from build123d import *

# Parameters (mm, degrees)
SKETCH1_R           = 1.5
BOSS_EXTRUDE1_DEPTH = 0.5
SKETCH2_R           = 1.5
BOSS_EXTRUDE2_DEPTH = 0.5
BOSS_EXTRUDE6_DEPTH = 10.25


with BuildPart() as part:
    # Sketch1 → Boss-Extrude1 (new, symmetric)
    with BuildSketch(Plane(origin=(0, 0, 0), x_dir=(0, 0, -1), z_dir=(1, 0, 0))):
        Polygon((0, 0), (0, 6), (14, 6), (14, -0.7), (9.85, -1), (9.7, 0), align=None)
        with Locations((10.4, 4)):
            Circle(SKETCH1_R, mode=Mode.SUBTRACT)
    extrude(amount=BOSS_EXTRUDE1_DEPTH, both=True)



with BuildPart() as body_2:
    # Sketch2 → Boss-Extrude2 (new, symmetric)
    with BuildSketch(Plane.ZY.offset(11.5)):
        Polygon((-9.7, 0), (-9.85, -1), (-14, -0.7), (-14, 6), (0, 6), (0, 0), align=None)
        with Locations(Location((-10.4, 4, 0), (0, 0, 180))):
            Circle(SKETCH2_R, mode=Mode.SUBTRACT)
    extrude(amount=BOSS_EXTRUDE2_DEPTH, both=True)


with BuildPart() as part_1:
    add(part.part)

    add(body_2.part)  # Boss-Extrude6 merges body 2
    # Sketch9 → Boss-Extrude6 (add)
    with BuildSketch(Plane.XY):
        with BuildLine():
            Line((-11, 6), (-12, 6))
            ThreePointArc((-12, 6), (-11.414213562, 7.414213562), (-10, 8))
            Line((-10, 8), (-1.5, 8))
            ThreePointArc((-1.5, 8), (-0.085786438, 7.414213562), (0.5, 6))
            Line((0.5, 6), (-0.5, 6))
            ThreePointArc((-0.5, 6), (-0.792893219, 6.707106781), (-1.5, 7))
            Line((-1.5, 7), (-10, 7))
            ThreePointArc((-10, 7), (-10.707106781, 6.707106781), (-11, 6))
        make_face()
    extrude(amount=-BOSS_EXTRUDE6_DEPTH)


solid = part_1.part
Input: part model. Units: mm. Frame: model coordinates. A direction names the side the tool comes from. Round coordinates to 2 decimals unless told otherwise and drop trailing zeros. Loops run counter-clockwise (first coordinate to the right, second up) from the corner with the lowest first, then second, coordinate; pieces in that order, holes last. Notation, with made-up numbers: (-6.5, 19.25) -> (-1.5, 19.25) arc R12 ccw to (-1.5, 40.25) -> close; hole circle Ø10 at (28, 28). An arc over 180 degrees is marked (long way). Answer as a JSON object with one key per item and string values. Group by question number.
1) Reachability of faces 1 (the flat face through (-11.51, -0.85, -11.9)), 2 (the flat face through (-0.5, 3, -7)), 3 (the flat face through (0, 6, -12)), 4 (the flat face through (-11.5, 0, -4.8)) from +Z, -Z, +X, -X, +Y, -Y: full face, straight path, thin tool, end or side. Return the list, or none.
2) Section query A-A on y = 0.25. Output: boundary loops of the cut face in (x, z), plus the area to 3 significant figures.
3) Ray query, L1, parallel to Z at x = -11.4, y = 4; L2, parallel to X at y = 1.75, z = -7.75; L3, parallel to Y at x = -1.5, z = -2.75. Return the intervals inside material, ascending.
4) Pin query (flat end, axial travel): pin 1 (0.6 mm diameter, centred on x = -5, y = 7, fed in from -Z); pin 2 (0.8 mm diameter, centred on x = -11.5, z = -3.5, fed in from -Y); pin 3 (0.5 mm diameter, centred on x = 0, z = -12, fed in from +Y). Return the tip coordinate at first contact, or that it passes through.
5) Section query C-C on y = 4. Output: boundary loops of the cut face in (x, z), plus the area to 3 significant figures.
6) Section query B-B on z = -9.5. Output: boundary loops of the cut face in (x, y), plus the area to 3 significant figures.
7) Section query D-D on z = -2.5. Output: boundary loops of the cut face in (x, y).
8) Draft query along X for faces 5 (the flat face through (0.5, 3, -7)), 6 (the flat face through (0, 3, -14)), 7 (the flat face through (-11, 3, -7)). Return one class per face: +X half, -X half, draft (parallel to the pull), parting line (faces both ways), or undercut.
Reply:
{
 "1": {"face 1": "-Z, +X, -X, -Y", "face 2": "+Z, -Z, -Y", "face 3": "-Z, +X, -X, +Y", "face 4": "+Z, +X, -X, -Y"},
 "2": {"outline": "(-12, -14) -> (-11, -14) -> (-11, 0) -> (-12, 0) -> close; (-0.5, -14) -> (0.5, -14) -> (0.5, 0) -> (-0.5, 0) -> close", "area": "28.0 mm2"},
 "3": {"L1": "z = -14 to -11.9, -8.9 to 0", "L2": "x = -12 to -11, -0.5 to 0.5", "L3": "y = 7 to 8"},
 "4": {"pin 1": "stops at z = -10.25", "pin 2": "stops at y = 0", "pin 3": "stops at y = 6"},
 "5": {"outline": "(-12, -14) -> (-11, -14) -> (-11, -11.9) -> (-12, -11.9) -> close; (-12, -8.9) -> (-11, -8.9) -> (-11, 0) -> (-12, 0) -> close; (-0.5, -14) -> (0.5, -14) -> (0.5, -11.9) -> (-0.5, -11.9) -> close; (-0.5, -8.9) -> (0.5, -8.9) -> (0.5, 0) -> (-0.5, 0) -> close", "area": "22.0 mm2"},
 "6": {"outline": "(-12, 0) -> (-11, 0) -> (-11, 2.8) -> (-12, 2.8) -> close; (-12, 5.2) -> (-11, 5.2) -> (-11, 6) arc R1 cw to (-10, 7) -> (-1.5, 7) arc R1 cw to (-0.5, 6) -> (-0.5, 5.2) -> (0.5, 5.2) -> (0.5, 6) arc R2 ccw to (-1.5, 8) -> (-10, 8) arc R2 ccw to (-12, 6) -> close; (-0.5, 0) -> (0.5, 0) -> (0.5, 2.8) -> (-0.5, 2.8) -> close", "area": "20.4 mm2"},
 "7": {"outline": "(-12, 0) -> (-11, 0) -> (-11, 6) arc R1 cw to (-10, 7) -> (-1.5, 7) arc R1 cw to (-0.5, 6) -> (-0.5, 0) -> (0.5, 0) -> (0.5, 6) arc R2 ccw to (-1.5, 8) -> (-10, 8) arc R2 ccw to (-12, 6) -> close"},
 "8": {"face 5": "+X half", "face 6": "draft", "face 7": "undercut"}
}
